Design review of the part built by this model. Coordinates are the model's own, in mm. A direction names the side the tool comes from. Coordinates: 2 decimals unless noted, no trailing zeros. Loops run counter-clockwise (first coordinate to the right, second up) from the corner with the lowest first, then second, coordinate; pieces in that order, holes last. Notation, with made-up numbers: M 86,-16.5 L 106,-16.5 A21 ccw 106,-12.5 Z; hole C -15,76.25 d10. An arc over 180 degrees is marked long. Put each result on its own line as item: value. Start each with the question number.
(1) For faces 1 (the flat face through (-1, 0, 1)), 2 (the flat face through (-6, 1, 1)), 3 (the flat face through (-5, -3.024, 1)), list the 3-axis set-ups (+Z, -Z, +X, -X, +Y, -Y) from which the entire face can be reached by the end or side of a thin tool; tool diameter is ignored.
(2) Take a section at B-B, the plane z = 1.75. Give the boundary of the cut face in (x, y), then the cut area to 3 significant figures.
(3) The part is to be moulded in two halves that separate along X. For faces 4 (the flat face through (-4, -9, 0)), 5 (the flat face through (-8.5, -10, 1)), 6 (the flat face through (-6.939, -8, 1)), 7 (the flat face through (-6.179, -13.142, 0.986)), say which applies: +X half, -X half, draft (parallel to the pull), parting line (faces both ways), or undercut.
(4) Clearance check with flat-ended pins moving along their axes: pin 1 (4 mm diameter, centred on x = -7, y = -15.5, fed in from -Z); pin 2 (1 mm diameter, centred on x = -7.5, z = 1.5, fed in from +Y); pin 3 (1.2 mm diameter, centred on y = 1, z = 0.5, fed in from +X). State where each tip first meets the part, or that it passes through.
(5) For probe 1 along X at (y, z) = (-5.5, 1.4); probe 2 along X at (y, z) = (-9.25, 1.45) (3 decimals); probe 3 along X at (y, z) = (-2, 0.35), list the stretches that pass through material, from the lowest coordinate up. Write a range as [from, to].
(6) Take a section at A-A, the plane x = -5. Give the boundary of the cut face in (y, z), then the cut area to 3 significant figures.
(7) Take a section at C-C, the plane y = -11.5. Give the boundary of the cut face in (x, z), then the cut area to 3 significant figures.
(8) Take a section at D-D, the plane y = -18. Give the boundary of the cut face in (x, z).
```python
from build123d import *

# Parameters (mm, degrees)
BOSS_EXTRUDE1_DEPTH = 2


with BuildPart() as part:
    # Sketch1 → Boss-Extrude1 (new body)
    with BuildSketch(Plane.XY):
        Polygon((-8.5, 0), (-8.5, -20), (-5.47292158, -18.243071932), (0, 0), (-2.5, 0), (-2.5, 1.5), (-6, 1.5), (-6, 0), align=None)
        Polygon((-3.439362664, -4.523577139), (-5.439362664, -12.713119984), (-6.939362664, -13.583725808), (-6.939362664, -12.713119984), (-6.939362664, -11.713119984), (-6.939362664, -4.523577139), (-6.939362664, -3.023577139), (-3.439362664, -3.023577139), (-3.07304185, -3.023577139), align=None, mode=Mode.SUBTRACT)
    extrude(amount=BOSS_EXTRUDE1_DEPTH)


solid = part.part
```
Computed values:
1. face 1: +Z, -Z, +X, +Y
1. face 2: +Z, -Z, -X, +Y
1. face 3: +Z, -Z
2. outline: M -8.5,-20 L -5.47,-18.24 L 0,0 L -2.5,0 L -2.5,1.5 L -6,1.5 L -6,0 L -8.5,0 Z; hole M -6.94,-13.58 L -5.44,-12.71 L -3.07,-3.02 L -6.94,-3.02 Z
2. area: 86.4 mm^2
3. face 4: draft
3. face 5: -X half
3. face 6: undercut
3. face 7: undercut
4. pin 1: stops at z = 0
4. pin 2: stops at y = 0
4. pin 3: stops at x = -2.5
5. probe 1: x = [-8.5, -6.94], [-3.68, -1.65]
5. probe 2: x = [-8.5, -6.939], [-4.594, -2.775]
5. probe 3: x = [-8.5, -0.6]
6. outline: M -16.67,0 L -10.91,0 L -10.91,2 L -16.67,2 Z; M -3.02,0 L 1.5,0 L 1.5,2 L -3.02,2 Z
6. area: 20.6 mm^2
7. outline: M -8.5,0 L -6.94,0 L -6.94,2 L -8.5,2 Z; M -5.14,0 L -3.45,0 L -3.45,2 L -5.14,2 Z
7. area: 6.51 mm^2
8. outline: M -8.5,0 L -5.4,0 L -5.4,2 L -8.5,2 Z
